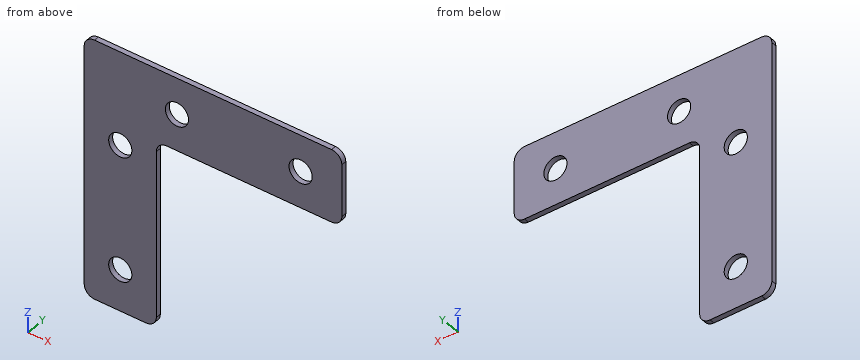
from build123d import *

# Parameters (mm, degrees)
SKETCH_1_R      = 2.25
EXTRUDE_2_DEPTH = 1


with BuildPart() as part:
    # 草图1 → 凸台-拉伸2 (new body)
    with BuildSketch(Plane(origin=(0, 0, 0), x_dir=(1, 0, 0), z_dir=(0, 1, 0))):
        with BuildLine():
            Line((2, 50), (12, 50))
            ThreePointArc((12, 50), (13.414213562, 49.414213562), (14, 48))
            Line((14, 48), (14, 16))
            ThreePointArc((14, 16), (14.585786438, 14.585786438), (16, 14))
            Line((16, 14), (48, 14))
            ThreePointArc((48, 14), (49.414213562, 13.414213562), (50, 12))
            Line((50, 12), (50, 2))
            ThreePointArc((50, 2), (49.414213562, 0.585786438), (48, 0))
            Line((48, 0), (2, 0))
            ThreePointArc((2, 0), (0.585786438, 0.585786438), (0, 2))
            Line((0, 2), (0, 48))
            ThreePointArc((0, 48), (0.585786438, 49.414213562), (2, 50))
        make_face()
        with Locations(Location((18, 7, 0), (0, 0, 270))):
            Circle(SKETCH_1_R, mode=Mode.SUBTRACT)
        with Locations(Location((42, 7, 0), (0, 0, 270))):
            Circle(SKETCH_1_R, mode=Mode.SUBTRACT)
        with Locations(Location((7, 18, 0), (0, 0, 270))):
            Circle(SKETCH_1_R, mode=Mode.SUBTRACT)
        with Locations(Location((7, 42, 0), (0, 0, 270))):
            Circle(SKETCH_1_R, mode=Mode.SUBTRACT)
    extrude(amount=EXTRUDE_2_DEPTH)


solid = part.part
Geometry: final body of the model. Coordinates: model frame, mm. Coordinates: 2 decimals unless noted, no trailing zeros. Loops run counter-clockwise (first coordinate to the right, second up) from the corner with the lowest first, then second, coordinate; pieces in that order, holes last. Notation, with made-up numbers: (76.5, -23) - (101.5, -23) arc R14 ccw to (101.5, -9) - close; hole circle Ø1 at (-4, 48). An arc over 180 degrees is marked (long way). One line per question, with ' | ' between items. Start each with the question number.
(1) Ray query, L1, parallel to X at y = 0.65, z = -7; L2, parallel to X at y = 0.85, z = -42; L3, parallel to X at y = 0.65, z = -38. Return the intervals inside material, ascending. Write a range as from..to.
(2) Cut plane B-B on y = 0.6. Output: boundary loops of the cut face in (x, z).
(3) Cut plane D-D on x = 42. Output: boundary loops of the cut face in (y, z).
(4) Cut plane C-C on z = -42. Output: boundary loops of the cut face in (x, y).
(5) First-contact query: pin 1 (4 mm diameter, centred on x = 7, z = -18, fed in from +Y); pin 2 (5 mm diameter, centred on x = 42, z = -7, fed in from +Y). Flat tips, straight axial feed; report the tip coordinate or a pass-through.
(6) Cut plane A-A on x = 7. Output: boundary loops of the cut face in (y, z).
Here are the results:
1) L1: 0..15.75, 20.25..39.75, 44.25..50 | L2: 0..4.75, 9.25..14 | L3: 0..14
2) outline: (0, -48) arc R2 ccw to (2, -50) - (12, -50) arc R2 ccw to (14, -48) - (14, -16) arc R2 cw to (16, -14) - (48, -14) arc R2 ccw to (50, -12) - (50, -2) arc R2 ccw to (48, 0) - (2, 0) arc R2 ccw to (0, -2) - close; hole circle Ø4.5 at (7, -42); hole circle Ø4.5 at (7, -18); hole circle Ø4.5 at (18, -7); hole circle Ø4.5 at (42, -7)
3) outline: (0, -14) - (1, -14) - (1, -9.25) - (0, -9.25) - close; (0, -4.75) - (1, -4.75) - (1, 0) - (0, 0) - close
4) outline: (0, 0) - (4.75, 0) - (4.75, 1) - (0, 1) - close; (9.25, 0) - (14, 0) - (14, 1) - (9.25, 1) - close
5) pin 1: through | pin 2: y = 1
6) outline: (0, -50) - (1, -50) - (1, -44.25) - (0, -44.25) - close; (0, -39.75) - (1, -39.75) - (1, -20.25) - (0, -20.25) - close; (0, -15.75) - (1, -15.75) - (1, 0) - (0, 0) - close
